Solid Edge part; units mm, degrees
sketch "Sketch1" plane through (0, 0, 0) normal (0, 0, -1) x (-1, 0, 0)
  line L0 (4, -46) -> (46, -4)
  line L1 (46, 0) -> (46, -4)
  line L2 (42, 0) -> (46, 0)
  line L3 (42, 6) -> (42, 0)
  line L4 (32, 6) -> (42, 6)
  line L5 (32, 0) -> (32, 6)
  line L6 (26.55, 0) -> (32, 0)
  line L7 (26.55, -2.5) -> (26.55, 0)
  line L8 (28, -2.5) -> (26.55, -2.5)
  line L9 (28, -5.5) -> (28, -2.5)
  line L10 (26.55, -5.5) -> (28, -5.5)
  line L11 (26.55, -13) -> (26.55, -5.5)
  line L12 (23.45, -13) -> (26.55, -13)
  line L13 (23.45, -5.5) -> (23.45, -13)
  line L14 (22, -5.5) -> (23.45, -5.5)
  line L15 (22, -2.5) -> (22, -5.5)
  line L16 (23.45, -2.5) -> (22, -2.5)
  line L17 (23.45, 0) -> (23.45, -2.5)
  line L18 (18, 0) -> (23.45, 0)
  line L19 (18, 0) -> (18, 6)
  line L20 (18, 6) -> (8, 6)
  line L21 (8, 6) -> (8, 0)
  line L22 (0, 0) -> (8, 0)
  line L23 (0, 0) -> (0, -8)
  line L24 (-6, -8) -> (0, -8)
  line L25 (-6, -18) -> (-6, -8)
  line L26 (-6, -18) -> (0, -18)
  line L27 (0, -18) -> (0, -23.45)
  line L28 (0, -23.45) -> (2.5, -23.45)
  line L29 (2.5, -23.45) -> (2.5, -22)
  line L30 (2.5, -22) -> (5.5, -22)
  line L31 (5.5, -22) -> (5.5, -23.45)
  line L32 (5.5, -23.45) -> (13, -23.45)
  line L33 (13, -23.45) -> (13, -26.55)
  line L34 (13, -26.55) -> (5.5, -26.55)
  line L35 (5.5, -26.55) -> (5.5, -28)
  line L36 (5.5, -28) -> (2.5, -28)
  line L37 (2.5, -28) -> (2.5, -26.55)
  line L38 (2.5, -26.55) -> (0, -26.55)
  line L39 (0, -26.55) -> (0, -32)
  line L40 (0, -32) -> (-6, -32)
  line L41 (-6, -32) -> (-6, -42)
  line L42 (-6, -42) -> (0, -42)
  line L43 (0, -42) -> (0, -46)
  line L44 (0, -46) -> (4, -46)
extrude "Protrusion1" add sketch "Sketch1" against normal blind 6
CAD build for the part. Positions are in the model's coordinates, mm. A direction names the side the tool comes from. Round coordinates to 2 decimals unless told otherwise and drop trailing zeros. Write each loop counter-clockwise with the first axis right and the second up, starting at its lowest first coordinate (ties: lowest second). Pieces come first, ordered by that corner, then holes.
Item 1: Drop flat-ended pins along their axis: pin 1 Ø3 at (y, z) = (3, 2) entering from +X; pin 2 Ø3 at (x, z) = (3.5, 2.5) entering from -Y; pin 3 Ø1.8 at (y, z) = (-8, 2) entering from -X. Give the stop position or say it passes through.
Filled in:
pin 1: stops at x = -8
pin 2: stops at y = -42
pin 3: stops at x = -42.9
Item 2: Band-saw the part on B-B on x = -33. Write the cut outline in (y, z).
Filled in:
outline: (-17, 0) - (6, 0) - (6, 6) - (-17, 6) - close
Item 3: Band-saw the part on A-A on y = -38.5. Write the cut outline in (x, z).
Filled in:
outline: (-11.5, 0) - (6, 0) - (6, 6) - (-11.5, 6) - close
Item 4: Tool access for faces 1 (the flat face through (-27, -2.5, 3)), 2 (the flat face through (-32, 3, 3)), 3 (the flat face through (3, -32, 3)): list every direction of +Z, -Z, +X, -X, +Y, -Y with a clear straight run to the whole face (end or side of a thin tool).
Filled in:
face 1: +Z, -Z
face 2: +Z, -Z, +Y
face 3: +Z, -Z, +X
Item 5: Mould opens along X. For faces 4 (the flat face through (6, -13, 3)), 5 (the flat face through (-5.5, -23, 3)), 6 (the flat face through (-2, -46, 3)) say: released by +X, released by -X, zero draft, split by the parting line, or undercut.
Filled in:
face 4: released by +X
face 5: undercut
face 6: zero draft
Item 6: Drill centre lines: L1, parallel to X at y = -4, z = 3.4; L2, parallel to Y at x = 0.5, z = 2.35; L3, parallel to X at y = -5, z = 3.7. Where is each one in solid material? Low to high.
Filled in:
L1: x = -46 to -28, -22 to 0
L2: y = -42 to -32, -18 to -8
L3: x = -45 to -28, -22 to 0
